Geometry check sheet. Reference: drawing and pictorial views, mm from the part's lowest x, y, z. A direction names the side the tool comes from. Give positions to 0.01 mm unless a question says otherwise; leave off trailing zeros. Write each loop counter-clockwise with the first axis right and the second up, starting at its lowest first coordinate (ties: lowest second). Pieces come first, ordered by that corner, then holes. Notation, with made-up numbers: (61.25, -6.5) -> (116.25, -6.5) arc R12 ccw to (116.25, 3.5) -> close; hole circle Ø8 at (-15, 74.25). An arc over 180 degrees is marked (long way). Answer as CSV lines item,"result".
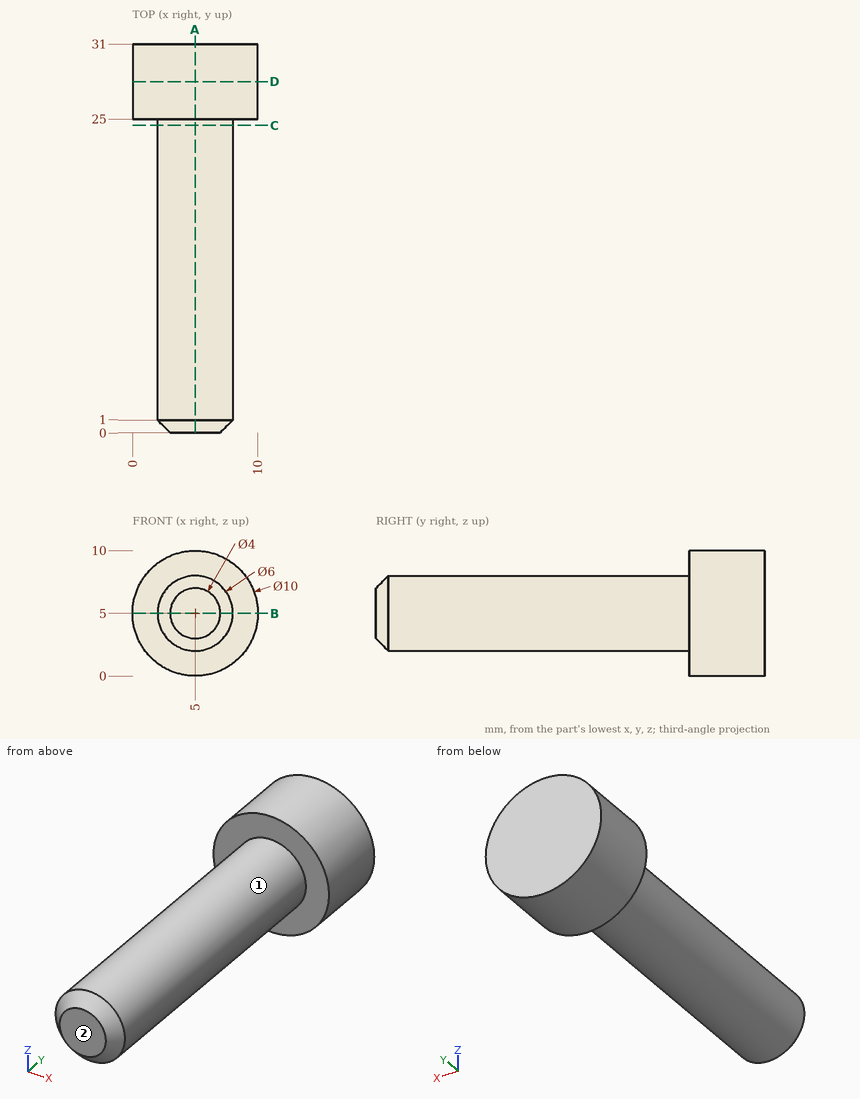
1) Tool access check on the marked faces 1 and 2. Record the directions out of +Z, -Z, +X, -X, +Y, -Y that give a thin tool (end or side, any length) a straight path to the whole face; none if there is none.
Reported:
face 1,"-Y"
face 2,"+Z, -Z, +X, -X, -Y"
2) Depth check by flat-ended pin: pin 1 (2 mm diameter, centred on y = 4.5, z = 8, fed in from +X); pin 2 (3 mm diameter, centred on x = 8, z = 3, fed in from -Y); pin 3 (1 mm diameter, centred on x = 4, y = 12, fed in from -Z). Enter the tip coordinate at first touch or a pass-through.
Reported:
pin 1,"x = 7.24"
pin 2,"y = 0.11"
pin 3,"z = 2.04"
3) Section check D-D (y = 28). Record the boundary of the cut face in (x, z).
Reported:
outline,"circle Ø10 at (5, 5)"
4) Section check C-C (y = 24.5). Record the boundary of the cut face in (x, z).
Reported:
outline,"circle Ø6 at (5, 5)"
5) Section check B-B (z = 5). Record the boundary of the cut face in (x, y).
Reported:
outline,"(0, 25) -> (2, 25) -> (2, 1) -> (3, 0) -> (7, 0) -> (8, 1) -> (8, 25) -> (10, 25) -> (10, 31) -> (0, 31) -> close"
6) Scan lines: line 1 along Y through (x, z) = (1.25, 2); line 2 along Y through (x, z) = (2.5, 3.5); line 3 along Z through (x, y) = (2.75, 5.5). Record each from-to range of solid material in increasing order.
Reported:
line 1,"25 to 31"
line 2,"0.92 to 31"
line 3,"3.02 to 6.98"
7) Section check A-A (x = 5). Record the boundary of the cut face in (y, z), and give its area (3 significant figures).
Reported:
outline,"(0, 3) -> (1, 2) -> (25, 2) -> (25, 0) -> (31, 0) -> (31, 10) -> (25, 10) -> (25, 8) -> (1, 8) -> (0, 7) -> close"
area,"209 mm²"
